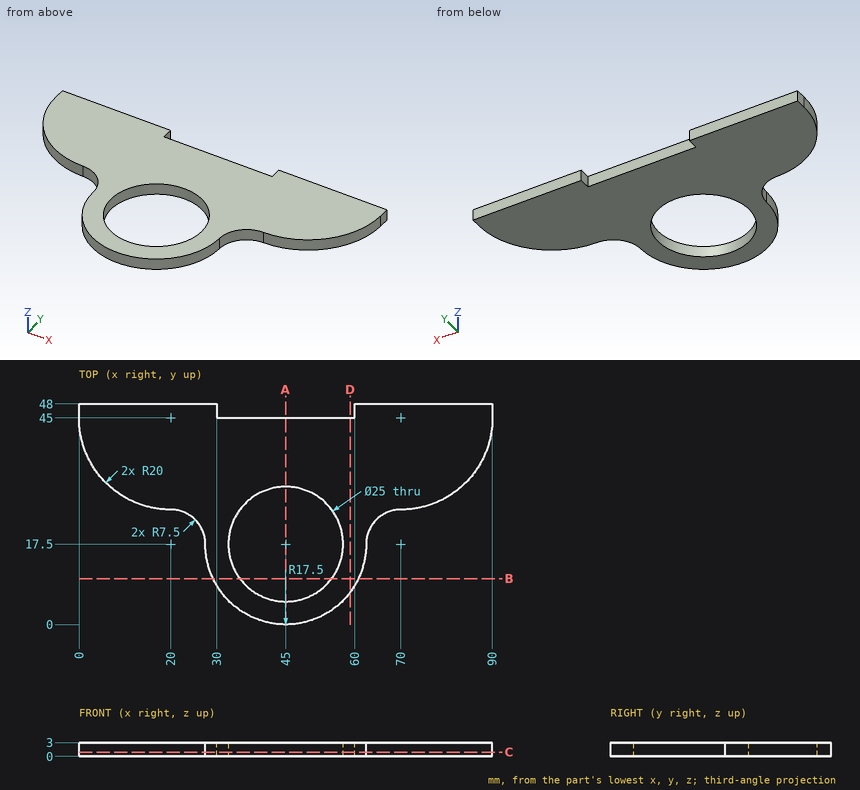
Here's the drawing with two shaded views (mm, measured from the low corner). I have some questions. Give positions to 0.01 mm unless a question says otherwise; leave off trailing zeros. Write each loop counter-clockwise with the first axis right and the second up, starting at its lowest first coordinate (ties: lowest second). Pieces come first, ordered by that corner, then holes. Notation, with made-up numbers: (0.5, 51) - (22.5, 51) arc R19 cw to (22.5, 77) - close; hole circle Ø9 at (0.5, 13.5). An arc over 180 degrees is marked (long way). Write item = value, one per line. Start each with the question number.
1. Please list where these lines run through material, in increasing order: line 1 (Y direction, x = 45, z = 0.75); line 2 (X direction, y = 46, z = 0.7); line 3 (X direction, y = 24, z = 2.7).
2. Imagine slicing it at D-D (x = 59). Please give me the cut outline in (y, z), and give its area (3 significant figures).
3. For pin 1 (15 mm diameter, centred on x = 45, y = 17.5, fed in from +Z) (3 decimals); pin 2 (1.5 mm diameter, centred on x = 17.5, z = 2, fed in from -Y); pin 3 (1.5 mm diameter, centred on x = 52.5, z = 1.5, fed in from +Y), each with a flat end and sliding along its axis, tell me the tip position at first contact or that it passes through.
4. Imagine slicing it at B-B (y = 10). Please give me the cut outline in (x, z), and give its area (3 significant figures).
5. Imagine slicing it at C-C (z = 0.9). Please give me the cut outline in (x, y), and give its area (3 significant figures).
6. Imagine slicing it at A-A (x = 45). Please give me the cut outline in (y, z), and give its area (3 significant figures).
Worked answers:
q1.line_1 = 0 to 5, 30 to 45
q1.line_2 = 0 to 30, 60 to 90
q1.line_3 = 23.74 to 34.32, 55.68 to 66.26
q2.outline = (7, 0) - (45, 0) - (45, 3) - (7, 3) - close
q2.area = 114 mm2
q3.pin_1 = through
q3.pin_2 = 25.08
q3.pin_3 = 45
q4.outline = (29.19, 0) - (35, 0) - (35, 3) - (29.19, 3) - close; (55, 0) - (60.81, 0) - (60.81, 3) - (55, 3) - close
q4.area = 34.9 mm2
q5.outline = (0, 45) arc R20 ccw to (20, 25) arc R7.5 cw to (27.5, 17.5) arc R17.5 ccw to (62.5, 17.5) arc R7.5 cw to (70, 25) arc R20 ccw to (90, 45) - (90, 48) - (60, 48) - (60, 45) - (30, 45) - (30, 48) - (0, 48) - close; hole circle Ø25 at (45, 17.5)
q5.area = 2,090 mm2
q6.outline = (0, 0) - (5, 0) - (5, 3) - (0, 3) - close; (30, 0) - (45, 0) - (45, 3) - (30, 3) - close
q6.area = 60.0 mm2
